```python
from build123d import *

# Parameters (mm, degrees)
F0_W           = 50
F0_H           = 50
F1_DEPTH       = 50
F3_D           = 10
F3_DEPTH       = 30
F3_CBORE_D     = 15
F3_CBORE_DEPTH = 10
F3_TIP         = 3.0043030951
F4_D           = 10
F4_DEPTH       = 30
F4_CBORE_D     = 15
F4_CBORE_DEPTH = 10
F4_TIP         = 3.0043030951
F5_W           = 62.9621855915
F5_H           = 46.8907589093
F6_DEPTH       = 20


with BuildPart() as f1:
    # F0 (on Top) → F1 (new body)
    with BuildSketch(Plane.XY):
        with Locations((-26.9832524723, 2.7374359779)):
            Rectangle(F0_W, F0_H)
    extrude(amount=F1_DEPTH)

    # F3
    with Locations(Plane.XY.offset(50)):
        with Locations((-31.9832524723, -2.2625640221)):
            CounterBoreHole(F3_D / 2, F3_CBORE_D / 2, F3_CBORE_DEPTH, depth=F3_DEPTH)
            with Locations((0, 0, -(F3_DEPTH + F3_TIP / 2))):  # 118° drill point
                Cone(0, F3_D / 2, F3_TIP, mode=Mode.SUBTRACT)

    # F4
    with Locations(Plane.XY.offset(50)):
        with Locations((-9.8126017437, 17.8528092922)):
            CounterBoreHole(F4_D / 2, F4_CBORE_D / 2, F4_CBORE_DEPTH, depth=F4_DEPTH)
            with Locations((0, 0, -(F4_DEPTH + F4_TIP / 2))):  # 118° drill point
                Cone(0, F4_D / 2, F4_TIP, mode=Mode.SUBTRACT)

    # F5 (on face) → F6 (cut)
    with BuildSketch(Plane.XZ.offset(22.2625640221)):
        with Locations((-22.54726924, 12.6207987778)):
            Rectangle(F5_W, F5_H)
    extrude(amount=-F6_DEPTH, mode=Mode.SUBTRACT)


solid = f1.part
```
For this review, take the finished solid that the model builds, in its own axes (mm). A direction names the side the tool comes from. Round coordinates to 2 decimals unless told otherwise and drop trailing zeros. Write each loop counter-clockwise with the first axis right and the second up, starting at its lowest first coordinate (ties: lowest second). Pieces come first, ordered by that corner, then holes.
1) Take a section at D-D on z = 43.5. Give the boundary of the cut face in (x, y), then the cut area to 3 significant figures.
Answer below:
outline: (-51.98, -22.26) - (-1.98, -22.26) - (-1.98, 27.74) - (-51.98, 27.74) - close; hole circle Ø15 at (-31.98, -2.26); hole circle Ø15 at (-9.81, 17.85)
area: 2,150 mm2
2) Take a section at B-B on z = 25. Give the boundary of the cut face in (x, y).
Answer below:
outline: (-51.98, -2.26) - (-36.98, -2.26) arc R5 cw to (-26.98, -2.26) - (-1.98, -2.26) - (-1.98, 27.74) - (-51.98, 27.74) - close; hole circle Ø10 at (-9.81, 17.85)
3) Take a section at A-A on y = -3. Give the boundary of the cut face in (x, z), then the cut area to 3 significant figures.
Answer below:
outline: (-51.98, 36.07) - (-36.93, 36.07) - (-36.93, 40) - (-39.45, 40) - (-39.45, 50) - (-51.98, 50) - close; (-27.04, 36.07) - (-1.98, 36.07) - (-1.98, 50) - (-24.52, 50) - (-24.52, 40) - (-27.04, 40) - close
area: 509 mm2
4) Insertion check: pin 1 Ø4 at (x, y) = (-25.5, -6) entering from -Z; pin 2 Ø4 at (x, z) = (-21.5, 13) entering from -Y; pin 3 Ø12 at (x, y) = (-31.98, -2.26) entering from +Z. Each pin has a flat end and moves straight along its axis. Give the tip position at first contact, or say it passes through.
Answer below:
pin 1: stops at z = 36.07
pin 2: stops at y = -2.26
pin 3: stops at z = 40
5) Mouldability with a two-part tool opening along Y and no side actions: class faces 1 (the face through (-27, 9, 50)), 2 (the face through (-6.35, 11.2, 45.07)), 3 (the face through (-27, -2.263, 18)) as +Y half, -Y half, draft (parallel to the pull), parting line (faces both ways), or undercut.
Answer below:
face 1: draft
face 2: undercut
face 3: -Y half
6) Machinability: for faces 4 (the face through (-31.94, -0.284, 18.185)), 5 (the face through (-27, -12, 36.066)), 6 (the face through (-6.1, 21.2, 29.9)), which of the approach directions +Z, -Z, +X, -X, +Y, -Y give a long, thin tool a straight path to every point of the face, cutting with its end or side? Answer none if there is none.
Answer below:
face 4: +Z, -Y
face 5: -Z, +X, -X, -Y
face 6: +Z
7) Take a section at C-C on x = -38.5. Give the boundary of the cut face in (y, z), then the cut area to 3 significant figures.
Answer below:
outline: (-22.26, 36.07) - (-2.26, 36.07) - (-2.26, 0) - (27.74, 0) - (27.74, 50) - (1.45, 50) - (1.45, 40) - (-5.97, 40) - (-5.97, 50) - (-22.26, 50) - close
area: 1,700 mm2
8) For line 1 along Y through (x, z) = (-18, 10); line 2 along Z through (x, y) = (-42, -14); line 3 along Y through (x, z) = (-30.5, 43), list the stretches that pass through material, from the lowest coordinate up.
Answer below:
line 1: y = -2.26 to 27.74
line 2: z = 36.07 to 50
line 3: y = -22.26 to -9.61, 5.09 to 27.74
